Verification items for this drawing (mm, ordinates from the low corner). A direction names the side the tool comes from. Round coordinates to 2 decimals unless told otherwise and drop trailing zeros. Loops run counter-clockwise (first coordinate to the right, second up) from the corner with the lowest first, then second, coordinate; pieces in that order, holes last. Notation, with made-up numbers: (26.25, 44) -> (32.25, 44) arc R15 ccw to (32.25, 71) -> close; hole circle Ø9 at (58, 32.25). An arc over 180 degrees is marked (long way). Use a Markdown table: item, result. Add a question column.
Q1. Sectioned sample at A-A, the plane y = 1.2. Enter the section's corners in (x, z), then the cut area to 3 significant figures.
Q2. Material ranges on L1, parallel to Z at x = 5, y = 1.65; L2, parallel to Z at x = 6.25, y = 1.9; L3, parallel to X at y = 0.8, z = 5, recorded low to high.
Q3. Gauge pin test, flat ends, axial feed: P1, Ø0.9, axis at x = 13, y = 2, coming from the -Z side; P2, Ø0.9, axis at y = 1, z = 12, coming from the +X side; P3, Ø0.9, axis at x = 13, y = 2, coming from the +Z side. Record the tip position at first contact, or that the pin passes through.
Q4. Sectioned sample at B-B, the plane z = 17.5. Enter the section's corners in (x, y).
Q5. Release check for a two-part mould opening along X. For the marked faces 1, 2 and 3 record: released by +X, released by -X, zero draft, split by the parting line, or undercut.
Q6. Set-up check for the marked faces 4, 5 and 6: record each of +Z, -Z, +X, -X, +Y, -Y from which the full face is reachable in a straight line by a thin tool's end or side.
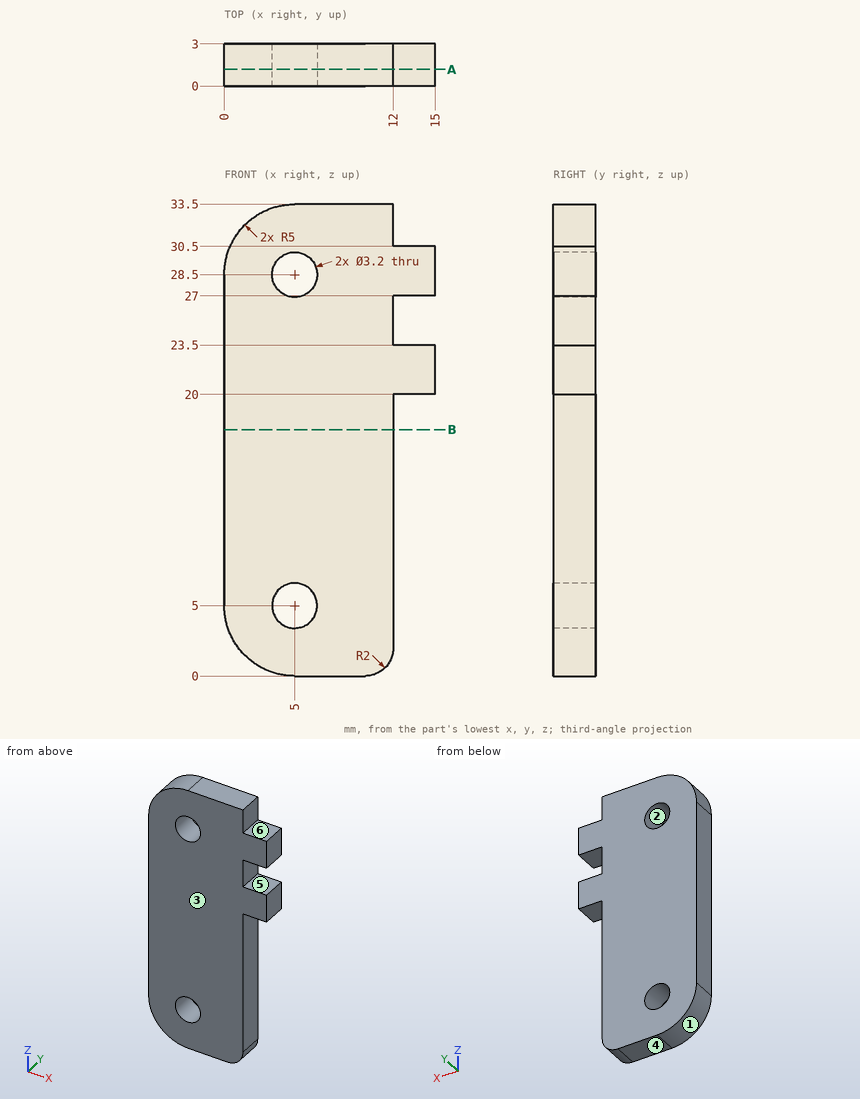
Values:
| question | item | result |
|---|---|---|
| 1 | outline | (0, 5) arc R5 ccw to (5, 0) -> (10, 0) arc R2 ccw to (12, 2) -> (12, 20) -> (15, 20) -> (15, 23.5) -> (12, 23.5) -> (12, 27) -> (15, 27) -> (15, 30.5) -> (12, 30.5) -> (12, 33.5) -> (5, 33.5) arc R5 ccw to (0, 28.5) -> close; hole circle Ø3.2 at (5, 5); hole circle Ø3.2 at (5, 28.5) |
| 1 | area | 395 mm^2 |
| 2 | L1 | 0 to 3.4, 6.6 to 26.9, 30.1 to 33.5 |
| 2 | L2 | 0 to 4, 6 to 27.5, 29.5 to 33.5 |
| 2 | L3 | 0 to 3.4, 6.6 to 12 |
| 3 | P1 | z = 20 |
| 3 | P2 | x = 12 |
| 3 | P3 | z = 30.5 |
| 4 | outline | (0, 0) -> (12, 0) -> (12, 3) -> (0, 3) -> close |
| 5 | face 1 | released by -X |
| 5 | face 2 | undercut |
| 5 | face 3 | zero draft |
| 6 | face 4 | -Z, +X, -X, +Y, -Y |
| 6 | face 5 | +X, +Y, -Y |
| 6 | face 6 | +Z, +X, +Y, -Y |
